```python
from build123d import *

# Parameters (mm, degrees)
SKETCH1_W           = 63.5
SKETCH1_H           = 50.8
BOSS_EXTRUDE1_DEPTH = 127
SKETCH2_W           = 31.75
SKETCH2_H           = 76.2
CUT_EXTRUDE1_DEPTH  = 50.8
CUT_EXTRUDE3_DEPTH  = 82.55
SKETCH4_W           = 31.75
SKETCH4_H           = 76.2
CUT_EXTRUDE4_DEPTH  = 63.5
CUT_EXTRUDE5_DEPTH  = 76.2
SKETCH6_R           = 4.7625
CUT_EXTRUDE6_DEPTH  = 503.011578552


with BuildPart() as part:
    # Sketch1 → Boss-Extrude1 (new body)
    with BuildSketch(Plane.XY):
        Polygon((63.5, -425.45), (63.5, 425.45), (31.75, 425.45), (31.75, 374.65), (-31.75, 374.65), (-31.75, 425.45), (-63.5, 425.45), (-63.5, -425.45), align=None)
        with Locations((0, 400.05)):
            Rectangle(SKETCH1_W, SKETCH1_H)
        with Locations((0, 450.85)):
            Rectangle(SKETCH1_W, SKETCH1_H)
    extrude(amount=BOSS_EXTRUDE1_DEPTH)

    # Sketch2 → Cut-Extrude1 (cut)
    with BuildSketch(Plane(origin=(63.5, 0, 0), x_dir=(0, 0, -1), z_dir=(1, 0, 0))):
        with Locations((-79.375, -260.35)):
            Rectangle(SKETCH2_W, SKETCH2_H)
    extrude(amount=-CUT_EXTRUDE1_DEPTH, mode=Mode.SUBTRACT)

    # Sketch3 → Cut-Extrude3 (cut)
    with BuildSketch(Plane.XY.offset(127)):
        with BuildLine():
            ThreePointArc((42.8625, -279.4), (41.467596045, -276.032403955), (38.1, -274.6375))
            Line((38.1, -274.6375), (38.1, -284.1625))
            ThreePointArc((38.1, -284.1625), (41.467596045, -282.767596045), (42.8625, -279.4))
        make_face()
        with BuildLine():
            Line((38.1, -284.1625), (38.1, -274.6375))
            ThreePointArc((38.1, -274.6375), (33.3375, -279.4), (38.1, -284.1625))
        make_face()
        with BuildLine():
            ThreePointArc((42.8625, -241.3), (41.467596045, -237.932403955), (38.1, -236.5375))
            Line((38.1, -236.5375), (38.1, -246.0625))
            ThreePointArc((38.1, -246.0625), (41.467596045, -244.667596045), (42.8625, -241.3))
        make_face()
        with BuildLine():
            Line((38.1, -246.0625), (38.1, -236.5375))
            ThreePointArc((38.1, -236.5375), (33.3375, -241.3), (38.1, -246.0625))
        make_face()
    extrude(amount=-CUT_EXTRUDE3_DEPTH, mode=Mode.SUBTRACT)

    # Sketch4 → Cut-Extrude4 (cut)
    with BuildSketch(Plane(origin=(0, 0, 0), x_dir=(-1, 0, 0), z_dir=(0, 0, -1))):
        with Locations((15.875, -260.35)):
            Rectangle(SKETCH4_W, SKETCH4_H)
    extrude(amount=-CUT_EXTRUDE4_DEPTH, mode=Mode.SUBTRACT)

    # Sketch5 → Cut-Extrude5 (cut)
    with BuildSketch(Plane.ZY.offset(63.5)):
        with BuildLine():
            ThreePointArc((31.75, -236.5375), (26.9875, -241.3), (31.75, -246.0625))
            Line((31.75, -246.0625), (31.75, -236.5375))
        make_face()
        with BuildLine():
            Line((31.75, -236.5375), (31.75, -246.0625))
            ThreePointArc((31.75, -246.0625), (35.117596045, -244.667596045), (36.5125, -241.3))
            ThreePointArc((36.5125, -241.3), (35.117596045, -237.932403955), (31.75, -236.5375))
        make_face()
        with BuildLine():
            ThreePointArc((31.75, -274.6375), (26.9875, -279.4), (31.75, -284.1625))
            Line((31.75, -284.1625), (31.75, -274.6375))
        make_face()
        with BuildLine():
            Line((31.75, -274.6375), (31.75, -284.1625))
            ThreePointArc((31.75, -284.1625), (35.117596045, -282.767596045), (36.5125, -279.4))
            ThreePointArc((36.5125, -279.4), (35.117596045, -276.032403955), (31.75, -274.6375))
        make_face()
    extrude(amount=-CUT_EXTRUDE5_DEPTH, mode=Mode.SUBTRACT)

    # Sketch6 → Cut-Extrude6 (cut, through all)
    with BuildSketch(Plane(origin=(31.75, 0, 0), x_dir=(0, 0, -1), z_dir=(1, 0, 0))):
        with Locations(Location((-95.25, 450.85, 0), (0, 0, 90))):
            Circle(SKETCH6_R)
        with Locations(Location((-31.75, 450.85, 0), (0, 0, 90))):
            Circle(SKETCH6_R)
    extrude(amount=-CUT_EXTRUDE6_DEPTH, mode=Mode.SUBTRACT)


solid = part.part
```
The model under review builds one solid part; all positions refer to its coordinate system, in mm. A direction names the side the tool comes from. Coordinates: 2 decimals unless noted, no trailing zeros. Write each loop counter-clockwise with the first axis right and the second up, starting at its lowest first coordinate (ties: lowest second). Pieces come first, ordered by that corner, then holes.
1) Clearance check with flat-ended pins moving along their axes: pin 1 Ø15 at (y, z) = (452.5, 71.5) entering from -X; pin 2 Ø9.5 at (x, y) = (-21, -267) entering from -Z; pin 3 Ø16 at (y, z) = (-276.5, 84.5) entering from +X. State where each tip first meets the part, or that it passes through.
2) To check wall thickness, follow probe 1 along Z at (x, y) = (10, 450.85); probe 2 along Y at (x, z) = (38.5, 98.5); probe 3 along Z at (x, y) = (10, 450). State the ranges of each line that lie inside material, in increasing order.
3) We need section C-C on z = 71. State the section outline as (x, y) points.
4) Machinability: for faces 5 (the face through (0, -261, 31)), 6 (the face through (63.5, -6, 63)), 7 (the face through (48, 425.45, 63)), 8 (the face through (38, -261, 95.25)), 9 (the face through (-31.75, 450, 63)), which of the approach directions +Z, -Z, +X, -X, +Y, -Y give a long, thin tool a straight path to every point of the face, cutting with its end or side? Answer none if there is none.
5) We need section A-A on x = -18. Count the separate pieces of the cut face and the enclosed holes in it, then the cut area to 3 significant figures.
6) The part is to be moulded in two halves that separate along X. For faces 1 (the face through (-16, -260, 63.5)), 2 (the face through (12.7, -260, 80)), 3 (the face through (-1, 32, 127)), 4 (the face through (-16, -298.45, 31)), say which applies: pulls with the +X half, pulls with the -X half, needs draft (parallel to the pull), parting line crosses it, or undercut.
Answer list:
1. pin 1: stops at x = -31.75
1. pin 2: stops at z = 63.5
1. pin 3: stops at x = 12.7
2. probe 1: z = 0 to 26.99, 36.51 to 90.49, 100.01 to 127
2. probe 2: y = -425.45 to -284.15, -274.65 to -246.05, -236.55 to 425.45
2. probe 3: z = 0 to 27.06, 36.44 to 90.56, 99.94 to 127
3. outline: (-63.5, -425.45) - (63.5, -425.45) - (63.5, -298.45) - (12.7, -298.45) - (12.7, -222.25) - (63.5, -222.25) - (63.5, 425.45) - (31.75, 425.45) - (31.75, 476.25) - (-31.75, 476.25) - (-31.75, 425.45) - (-63.5, 425.45) - close
4. face 5: -Z
4. face 6: +Z, -Z, +X, +Y, -Y
4. face 7: +Z, -Z, +X, +Y
4. face 8: +X
4. face 9: +Z, -Z, -X, +Y
5. separate pieces: 1
5. enclosed holes: 2
5. area: 110,000 mm2
6. face 1: undercut
6. face 2: pulls with the +X half
6. face 3: needs draft
6. face 4: undercut
